CAD build for the part. Positions are in the model's coordinates, mm. Round coordinates to 2 decimals unless told otherwise and drop trailing zeros. Order: outer loops, then holes, each group sorted by start corner. A loop starts at its lowest first (then second) coordinate and runs counter-clockwise, first axis right, second up. Notation, with made-up numbers: M -12.75,35.5 L 8.25,35.5 A33 cw 8.25,66.5 Z; hole C -18.5,65 d3. An arc over 180 degrees is marked long. Answer as CSV lines item,"result". Start each with the question number.
```python
from build123d import *

# Parameters (mm, degrees)
SKETCH2_R              = 10.387693019
SKETCH2_R_2            = 9.525
BOSS_EXTRUDE1_DEPTH    = 1.5875
F_10_CLEARANCE_HOLE1_D = 4.9784


with BuildPart() as part:
    # Sketch2 → Boss-Extrude1 (new body)
    with BuildSketch(Plane.XY):
        with BuildLine():
            Line((25.091057906, -52.092444741), (-65.683756135, -78.000081372))
            ThreePointArc((-65.683756135, -78.000081372), (-92.150845981, -65.52313309), (-83.314246567, -37.628768173))
            Line((-83.314246567, -37.628768173), (5.271270971, 16.133758159))
            ThreePointArc((5.271270971, 16.133758159), (13.983534085, 19.911144202), (23.391278089, 21.202084415))
            Line((23.391278089, 21.202084415), (37.879087429, 21.202084415))
            ThreePointArc((37.879087429, 21.202084415), (39.136323286, 21.722848558), (39.657087429, 22.980084415))
            Line((39.657087429, 22.980084415), (39.657087429, 23.085322173))
            ThreePointArc((39.657087429, 23.085322173), (46.007087429, 29.435322173), (52.357087429, 23.085322173))
            Line((52.357087429, 23.085322173), (52.357087429, 22.980084415))
            ThreePointArc((52.357087429, 22.980084415), (52.877851572, 21.722848558), (54.135087429, 21.202084415))
            Line((54.135087429, 21.202084415), (59.957258632, 21.202084415))
            ThreePointArc((59.957258632, 21.202084415), (63.54936108, 19.714186863), (65.037258632, 16.122084415))
            Line((65.037258632, 16.122084415), (65.037258632, -20.861923216))
            ThreePointArc((65.037258632, -20.861923216), (64.543779313, -23.046008387), (63.159216098, -24.805762511))
            Line((63.159216098, -24.805762511), (37.51946621, -45.622378614))
            ThreePointArc((37.51946621, -45.622378614), (31.63306192, -49.487085384), (25.091057906, -52.092444741))
        make_face()
        with Locations((15.016809712, -18.883068303)):
            Circle(SKETCH2_R, mode=Mode.SUBTRACT)
        with Locations((-72.258332946, -56.628468385)):
            Circle(SKETCH2_R_2, mode=Mode.SUBTRACT)
    extrude(amount=BOSS_EXTRUDE1_DEPTH)

    # #10 Clearance Hole1 (through all)
    with Locations(Plane.XY.offset(1.5875)):
        with Locations((-56.041369259, -27.019222928), (-8.951277081, -51.090630662), (46.007087429, 23.085322173)):
            Hole(F_10_CLEARANCE_HOLE1_D / 2)


solid = part.part
```
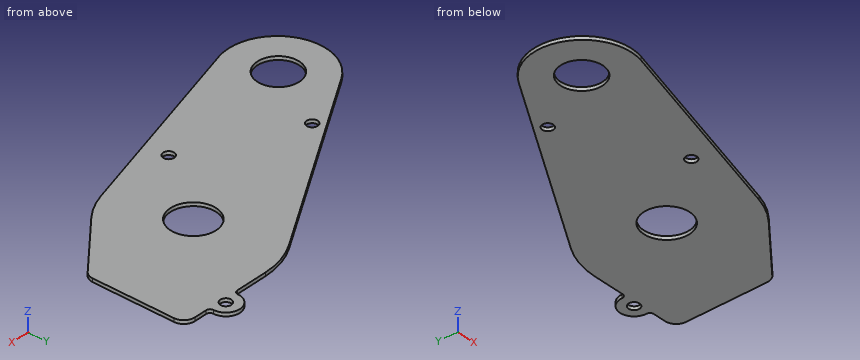
Q1. Band-saw the part on D-D, the plane y = 7. Write the cut outline in (x, z).
Q2. Band-saw the part on B-B, the plane x = -77. Write the cut outline in (y, z).
Q3. Drop a flat-ended pin along its axis: P1, Ø0.8, axis at x = 31, z = 1, coming from the +Y side. Give the stop position or say it passes through.
Q4. Probe line 1 along X through (y, z) = (-50, 0.7); line 2 along Y through (x, z) = (-64, 0.2); line 3 along Y through (x, z) = (-74.5, 0.85). List the from-to ranges inside material, lowest first. Write a range as from..to.
Q5. Band-saw the part on A-A, the plane y = -62. Write the cut outline in (x, z).
Q6. Band-saw the part on C-C, the plane z = 0.55. Count the separate pieces of the cut face and the enclosed holes in it, then the cut area to 3 significant figures.
Answer:
1,outline,"M -9.78,0 L 65.04,0 L 65.04,1.59 L -9.78,1.59 Z"
2,outline,"M -78.23,0 L -64.89,0 L -64.89,1.59 L -78.23,1.59 Z; M -48.37,0 L -33.8,0 L -33.8,1.59 L -48.37,1.59 Z"
3,P1,"stops at y = 21.2"
4,line 1,"x = -93..-79.1, -65.42..-11.19, -6.71..30.61"
4,line 2,"y = -77.52..-61.37, -51.88..-25.91"
4,line 3,"y = -78.69..-65.89, -47.37..-32.28"
5,outline,"M -93.35,0 L -80.12,0 L -80.12,1.59 L -93.35,1.59 Z; M -64.39,0 L -9.62,0 L -9.62,1.59 L -64.39,1.59 Z"
6,separate pieces,"1"
6,enclosed holes,"5"
6,area,"8,820 mm^2"
